Part model, mm, in its own coordinate system. A direction names the side the tool comes from. Give positions to 0.01 mm unless a question says otherwise; leave off trailing zeros. Write each loop counter-clockwise with the first axis right and the second up, starting at its lowest first coordinate (ties: lowest second). Pieces come first, ordered by that corner, then holes. Notation, with made-up numbers: M -28.5,-15.75 L -5.5,-15.75 A12 cw -5.5,7.25 Z; hole C 77,17.5 d10. An arc over 180 degrees is marked long. Use a Markdown table: item, result. Add a question column.
from build123d import *

# Parameters (mm, degrees)
F0_W         = 5
F0_H         = 2
F1_DEPTH     = 3
F2_R         = 2
F3_DEPTH     = 4
F4_W         = 219.5
F4_H         = 34
F4_W_2       = 214.53166008
F4_H_2       = 28.9933998138
F5_DEPTH     = 2
F6_R         = 2.5
F7_DEPTH     = 7.001
F8_R         = 5
F9_DEPTH     = 4
F10_W        = 13.5
F10_H        = 4
F11_DEPTH    = 25
F12_T1_DEPTH = 5


# Not quite as in the source:
# - a fillet or chamfer that OpenCascade refuses, or shapes differently, is made with other operations: its cross-section is extruded or revolved along the edge and cut away or added
# - a feature names something its author has since deleted; it is built from what else it names


with BuildPart() as f1:
    # F0 (on Front) → F1 (new body)
    with BuildSketch(Plane.XZ):
        Polygon((111.25, 5), (111.25, 18.75), (-111.25, 18.75), (-111.25, 5), (-111.25, -5), (-111.25, -18.75), (111.25, -18.75), (111.25, -5), align=None)
        with Locations((0, -12.25)):
            Rectangle(F0_W, F0_H, mode=Mode.SUBTRACT)
        with BuildLine():
            Line((-102, 12), (-8, 12))
            ThreePointArc((-8, 12), (-5.8786796564, 11.1213203436), (-5, 9))
            Line((-5, 9), (-5, -9))
            ThreePointArc((-5, -9), (-5.8786796564, -11.1213203436), (-8, -12))
            Line((-8, -12), (-102, -12))
            ThreePointArc((-102, -12), (-104.1213203436, -11.1213203436), (-105, -9))
            Line((-105, -9), (-105, 9))
            ThreePointArc((-105, 9), (-104.1213203436, 11.1213203436), (-102, 12))
        make_face(mode=Mode.SUBTRACT)
        with BuildLine():
            Line((8, 12), (102, 12))
            ThreePointArc((102, 12), (104.1213203436, 11.1213203436), (105, 9))
            Line((105, 9), (105, -9))
            ThreePointArc((105, -9), (104.1213203436, -11.1213203436), (102, -12))
            Line((102, -12), (8, -12))
            ThreePointArc((8, -12), (5.8786796564, -11.1213203436), (5, -9))
            Line((5, -9), (5, 9))
            ThreePointArc((5, 9), (5.8786796564, 11.1213203436), (8, 12))
        make_face(mode=Mode.SUBTRACT)
        with Locations((0, 12.25)):
            Rectangle(F0_W, F0_H, mode=Mode.SUBTRACT)
        with BuildLine():
            ThreePointArc((111.25, -5), (116.25, 0), (111.25, 5))
            Line((111.25, 5), (111.25, -5))
        make_face()
        with BuildLine():
            Line((-111.25, -5), (-111.25, 5))
            ThreePointArc((-111.25, 5), (-116.25, 0), (-111.25, -5))
        make_face()
    extrude(amount=F1_DEPTH)

    # F2 (on face) → F3 (join)
    with BuildSketch(Plane.XZ.offset(3)):
        with BuildLine():
            ThreePointArc((111.25, -5), (116.25, 0), (111.25, 5))
            Line((111.25, 5), (111.25, 18.75))
            Line((111.25, 18.75), (-111.25, 18.75))
            Line((-111.25, 18.75), (-111.25, 5))
            ThreePointArc((-111.25, 5), (-116.25, 0), (-111.25, -5))
            Line((-111.25, -5), (-111.25, -18.75))
            Line((-111.25, -18.75), (111.25, -18.75))
            Line((111.25, -18.75), (111.25, -5))
        make_face()
        with Locations((-111.25, 0)):
            Circle(F2_R, mode=Mode.SUBTRACT)
        with BuildLine():
            Line((-107.25, 15.75), (107.25, 15.75))
            ThreePointArc((107.25, 15.75), (107.9571067812, 15.4571067812), (108.25, 14.75))
            Line((108.25, 14.75), (108.25, -14.75))
            ThreePointArc((108.25, -14.75), (107.9571067812, -15.4571067812), (107.25, -15.75))
            Line((107.25, -15.75), (-107.25, -15.75))
            ThreePointArc((-107.25, -15.75), (-107.9571067812, -15.4571067812), (-108.25, -14.75))
            Line((-108.25, -14.75), (-108.25, 14.75))
            ThreePointArc((-108.25, 14.75), (-107.9571067812, 15.4571067812), (-107.25, 15.75))
        make_face(mode=Mode.SUBTRACT)
        with Locations((111.25, 0)):
            Circle(F2_R, mode=Mode.SUBTRACT)
    extrude(amount=F3_DEPTH)

    # F4 (on face) → F5 (cut)
    with BuildSketch(Plane.XZ.offset(7)):
        Rectangle(F4_W, F4_H)
        Rectangle(F4_W_2, F4_H_2, mode=Mode.SUBTRACT)
    extrude(amount=-F5_DEPTH, mode=Mode.SUBTRACT)

    # F6 (on face) → F7 (cut, through all)
    with BuildSketch(Plane.XZ.offset(7)):
        with Locations((-111.25, 0)):
            Circle(F6_R)
        with Locations((111.25, 0)):
            Circle(F6_R)
    extrude(amount=-F7_DEPTH, mode=Mode.SUBTRACT)

    # F8 (on face) → F9 (cut)
    with BuildSketch(Plane(origin=(0, 0, 0), x_dir=(-1, 0, 0), z_dir=(0, 1, 0))):
        with Locations((-111.25, 0)):
            Circle(F8_R)
        with Locations((111.25, 0)):
            Circle(F8_R)
    extrude(amount=-F9_DEPTH, mode=Mode.SUBTRACT)

    # F10 (on face) → F11 (cut)
    with BuildSketch(Plane(origin=(0, 0, -18.75), x_dir=(1, 0, 0), z_dir=(0, 0, -1))):
        with Locations((-55, 5)):
            Rectangle(F10_W, F10_H)
        with Locations((55, 5)):
            Rectangle(F10_W, F10_H)
    extrude(amount=-F11_DEPTH, mode=Mode.SUBTRACT)

    # F12: fillet of radius 3.5 on 2 edges, made by hand

    # F12_s2 → F12_t1 (cut)
    with BuildSketch(Plane.YZ.offset(-2.5)):
        with BuildLine():
            ThreePointArc((0, 7.7858983849), (-0.8542486889, 10.0771862323), (-3, 11.25))
            Line((-3, 11.25), (0, 11.25))
            Line((0, 11.25), (0, 7.7858983849))
        make_face()
        with BuildLine():
            ThreePointArc((0, -7.7858983849), (-0.8542486889, -10.0771862323), (-3, -11.25))
            Line((-3, -11.25), (0, -11.25))
            Line((0, -11.25), (0, -7.7858983849))
        make_face()
    extrude(amount=F12_T1_DEPTH, mode=Mode.SUBTRACT)


solid = f1.part
1. Cut at A-A (x = -23). Write the cut outline in (y, z).
2. Mould opens along X. For faces 1 (the flat face through (2, -3, 18.75)), 2 (the cylindrical face through (113.635, -5.521, 0.751)), 3 (the cylindrical face through (106.25, -1.97, -0.11)) say: released by +X, released by -X, zero draft, split by the parting line, or undercut.
3. Flat gauge pins, fed straight in: pin 1 (1.6 mm diameter, centred on y = -6.5, z = 9.5, fed in from -X); pin 2 (10.5 mm diameter, centred on x = 14.5, z = 4, fed in from -Y); pin 3 (0.6 mm diameter, centred on y = -4, z = -2, fed in from +X); pin 4 (1.6 mm diameter, centred on x = 51, y = -6.5, fed in from -Z). Where does each tip first touch, or does it go through?
4. Cut at C-C (y = -1.75). Give the number of separate pieces and of enclosed holes in the cut face, then the cut area to 3 significant figures.
5. Tool access for faces 4 (the flat face through (111.25, -3, -12)), 5 (the flat face through (-1, -5, 16)), 6 (the cylindrical face through (-106.25, -1.97, 0.11)), 7 (the flat face through (-111.25, -3, 12)), 8 (the flat face through (-111.25, -3, -12)): list every direction of +Z, -Z, +X, -X, +Y, -Y with a clear straight run to the whole face (end or side of a thin tool).
6. Drill centre lines: probe 1 along X at (y, z) = (-0.5, 7); probe 2 along Z at (x, y) = (88.5, -2.25); probe 3 along X at (y, z) = (-4, 10). Where is each one in solid material? Low to high. Write a range as [from, to].
7. Cut at B-B (z = 0). Write the cut outline in (x, y).
A:
| question | item | result |
|---|---|---|
| 1 | outline | M -7,-18.75 L 0,-18.75 L 0,-12 L -3,-12 L -3,-15.75 L -5,-15.75 L -5,-17 L -7,-17 Z; M -7,17 L -5,17 L -5,15.75 L -3,15.75 L -3,12 L 0,12 L 0,18.75 L -7,18.75 Z |
| 2 | face 1 | zero draft |
| 2 | face 2 | undercut |
| 2 | face 3 | released by +X |
| 3 | pin 1 | stops at x = -111.25 |
| 3 | pin 2 | passes through |
| 3 | pin 3 | stops at x = 115.95 |
| 3 | pin 4 | stops at z = 17 |
| 4 | separate pieces | 1 |
| 4 | enclosed holes | 4 |
| 4 | area | 3,460 mm² |
| 5 | face 4 | -Z, +X, +Y, -Y |
| 5 | face 5 | -Y |
| 5 | face 6 | -X, +Y |
| 5 | face 7 | +Z, -X, +Y, -Y |
| 5 | face 8 | -Z, -X, +Y, -Y |
| 6 | probe 1 | x = [-111.25, -105], [-5, 5], [105, 111.25] |
| 6 | probe 2 | z = [-18.75, -12], [12, 18.75] |
| 6 | probe 3 | x = [-111.25, -108.25], [108.25, 111.25] |
| 7 | outline | M -116.25,-7 L -113.75,-7 L -113.75,-4 L -116.25,-4 Z; M -108.75,-5 L -108.25,-5 L -108.25,-4 L -108.75,-4 Z; M -106.25,-3 L -105,-3 L -105,0 L -106.25,0 Z; M -5,-3 L 5,-3 L 5,0 L -5,0 Z; M 105,-3 L 106.25,-3 L 106.25,0 L 105,0 Z; M 108.25,-5 L 108.75,-5 L 108.75,-4 L 108.25,-4 Z; M 113.75,-7 L 116.25,-7 L 116.25,-4 L 113.75,-4 Z |
